Input: part model. Units: mm. Frame: model coordinates. Coordinates: 2 decimals unless noted, no trailing zeros. Write each loop counter-clockwise with the first axis right and the second up, starting at its lowest first coordinate (ties: lowest second). Pieces come first, ordered by that corner, then holes. Notation, with made-up numbers: (77, 40.5) - (121, 40.5) arc R16 ccw to (121, 49.5) - close; hole circle Ø5 at (61.5, 82.5). An arc over 180 degrees is marked (long way). One line per question, with ' | ' between items. Start each with the question number.
1) Line query: line 1 (Y direction, x = 2.85, z = 10); line 2 (Y direction, x = 2.9, z = 15); line 3 (Z direction, x = 2.95, y = 39). Output: solid intervals per line, ascending.
2) Section query D-D on z = 15.5. Return loops of the section in (x, y) (3 decimals).
3) Section query B-B on x = 1.95. Give the number of separate pieces and of enclosed holes in the cut face, and give its area (3 significant figures).
4) Section query C-C on y = 3. Return loops of the section in (x, z) (3 decimals), and give its area (3 significant figures).
5) Section query A-A on z = -38.1. Return loops of the section in (x, y) (3 decimals).
6) First-contact query: P1, Ø1, axis at x = 1, y = -52.5, coming from the +Z side; P2, Ø1, axis at x = 2, y = -29.5, coming from the -Z side; P3, Ø3.5, axis at y = -42.11, z = -38.1, coming from the +X side; P4, Ø1.6, axis at x = 1.5, z = -67.5, coming from the -Y side. Flat tips, straight axial feed; report the tip coordinate or a pass-through.
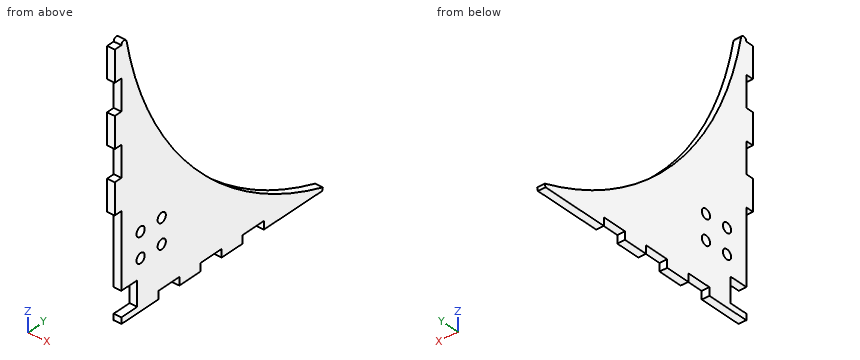
```python
from build123d import *

# Parameters (mm, degrees)
F0_W     = 3.175
F0_H     = 12.7
F0_R     = 1.984375
F1_DEPTH = 3.175


with BuildPart() as f1:
    # F0 (on Right) → F1 (new body)
    with BuildSketch(Plane.YZ):
        with Locations((-52.966131, 31.75)):
            Rectangle(F0_W, F0_H)
        with Locations((-52.966131, 6.35)):
            Rectangle(F0_W, F0_H)
        with Locations((-52.966131, -19.05)):
            Rectangle(F0_W, F0_H)
        with BuildLine():
            ThreePointArc((-48.86175, 38.34122), (-50.229793, 39.364207), (-51.378631, 38.1))
            Line((-51.378631, 38.1), (-51.378631, 25.4))
            Line((-51.378631, 25.4), (-51.378631, 12.7))
            Line((-51.378631, 12.7), (-51.378631, 0))
            Line((-51.378631, 0), (-51.378631, -12.7))
            Line((-51.378631, -12.7), (-51.378631, -25.4))
            Line((-51.378631, -25.4), (-51.378631, -55.88))
            Line((-51.378631, -55.88), (-43.758631, -55.88))
            Line((-43.758631, -55.88), (-43.758631, -66.04))
            Line((-43.758631, -66.04), (-51.378631, -66.04))
            Line((-51.378631, -66.04), (-51.378631, -68.58))
            Line((-51.378631, -68.58), (-33.598631, -68.58))
            Line((-33.598631, -68.58), (-33.598631, -65.278))
            Line((-33.598631, -65.278), (-23.438631, -65.278))
            Line((-23.438631, -65.278), (-23.438631, -68.58))
            Line((-23.438631, -68.58), (-13.278631, -68.58))
            Line((-13.278631, -68.58), (-13.278631, -65.278))
            Line((-13.278631, -65.278), (-3.118631, -65.278))
            Line((-3.118631, -65.278), (-3.118631, -68.58))
            Line((-3.118631, -68.58), (7.041369, -68.58))
            Line((7.041369, -68.58), (7.041369, -65.278))
            Line((7.041369, -65.278), (17.201369, -65.278))
            Line((17.201369, -65.278), (17.201369, -68.58))
            Line((17.201369, -68.58), (45.269527, -68.58))
            Line((45.269527, -68.58), (45.648292, -67.367797))
            ThreePointArc((45.648292, -67.367797), (-16.189845, -27.551447), (-48.86175, 38.34122))
        make_face()
        with Locations((-42.107631, -48.26)):
            Circle(F0_R, mode=Mode.SUBTRACT)
        with Locations((-31.947631, -48.26)):
            Circle(F0_R, mode=Mode.SUBTRACT)
        with Locations((-42.107631, -38.1)):
            Circle(F0_R, mode=Mode.SUBTRACT)
        with Locations((-31.947631, -38.1)):
            Circle(F0_R, mode=Mode.SUBTRACT)
    extrude(amount=F1_DEPTH)


solid = f1.part
```
Answer key:
1) line 1: -54.55 to -40.14 | line 2: -51.38 to -42.17 | line 3: -68.58 to -65.1
2) outline: (0, -51.379) - (3.175, -51.379) - (3.175, -42.366) - (0, -42.366) - close
3) separate pieces: 1 | enclosed holes: 4 | area: 3,400 mm²
4) outline: (0, -68.58) - (3.175, -68.58) - (3.175, -45.307) - (0, -45.307) - close | area: 73.9 mm²
5) outline: (0, -51.379) - (3.175, -51.379) - (3.175, -44.092) - (0, -44.092) - close; (0, -40.123) - (3.175, -40.123) - (3.175, -33.932) - (0, -33.932) - close; (0, -29.963) - (3.175, -29.963) - (3.175, -5.684) - (0, -5.684) - close
6) P1: z = 38.1 | P2: z = -65.28 | P3: through | P4: y = -51.38
